Can you work these out from the model? Positions are in its coordinate system, mm. Face numbers are marked on the shaded views. A direction names the side the tool comes from. Give positions to 0.01 mm unless a question says otherwise; leave off trailing zeros. Loops run counter-clockwise (first coordinate to the right, second up) from the corner with the lowest first, then second, coordinate; pieces in that order, holes last. Notation, with made-up numbers: (-39.5, 1) -> (-1.5, 1) arc R26 ccw to (-1.5, 39) -> close; hole circle Ø2 at (36.5, 17.25). An arc over 180 degrees is marked (long way). Return JSON: item names as keys, results as strings. Group by question number.
Q1. Suppose I cut it at B-B, the plane z = -5. Please give me the cut outline in (x, y).
Q2. Suppose I cut it at D-D, the plane x = -13.5. Please give me the cut outline in (y, z).
Q3. I need wall thicknesses on line 1 along Y through (x, z) = (-4, -3); line 2 along X through (y, z) = (-8.45, -5); line 3 along Z through (x, y) = (27.5, -3). Which ranges of each line are inside material? Lowest first, please. Write a range as [from, to].
Q4. Suppose I cut it at C-C, the plane y = -4.5. Please give me the cut outline in (x, z).
Q5. Which directions (+Z, -Z, +X, -X, +Y, -Y) give clear straight access to the entire face, cutting with the end or side of a thin tool? Please do the marked faces 1 and 2.
Q6. Suppose I cut it at A-A, the plane x = -50. Please give me the cut outline in (y, z).
Q7. Will these pins go through, and if not, where does the flat tip stop? pin 1 (1 mm diameter, centred on x = 32.5, z = -0.5, fed in from +Y); pin 2 (0.6 mm diameter, centred on x = 60, y = -0.5, fed in from +Z); pin 3 (2.5 mm diameter, centred on x = 0, z = -5, fed in from -Y); pin 4 (5 mm diameter, centred on y = -6, z = -2.5, fed in from +X).
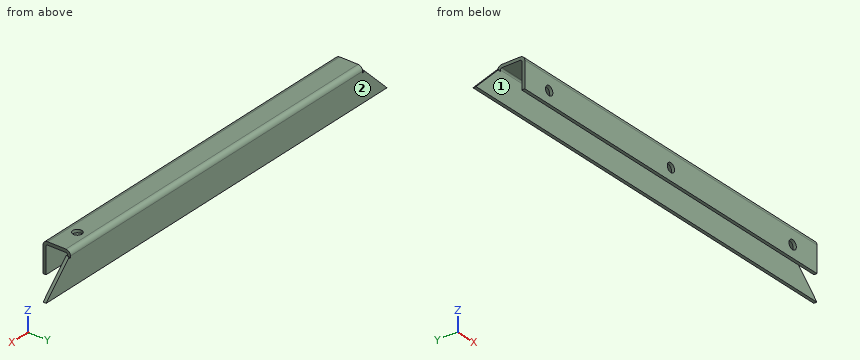
```python
from build123d import *

# Parameters (mm, degrees)
BASE_FLANGE1_DEPTH            = 1
EDGE_FLANGE1_STRIP_W          = 5
EDGE_FLANGE1_STRIP_H          = 1
EDGE_FLANGE1_STRIP_CUT_DEPTH  = 120
EDGE_FLANGE1_RELIEF_W         = 5.5
EDGE_FLANGE1_RELIEF_H         = 0.5
EDGE_FLANGE1_RELIEF_CUT_DEPTH = 1
EDGE_FLANGE1_DEPTH            = 120
EDGE_FLANGE2_STRIP_W          = 5
EDGE_FLANGE2_STRIP_H          = 1
EDGE_FLANGE2_STRIP_CUT_DEPTH  = 120
EDGE_FLANGE2_DEPTH            = 120
SKETCH12_R                    = 1.5
CUT_EXTRUDE1_DEPTH            = 3
SKETCH13_R                    = 1.5
CUT_EXTRUDE2_DEPTH            = 3


# Sheet-metal steps are written as plain solids
with BuildPart() as part:
    # Sketch1 → Base-Flange1 (new body)
    with BuildSketch(Plane(origin=(0, 0, 0), x_dir=(1, 0, 0), z_dir=(0, 1, 0))):
        Polygon((-60, 0), (60, 0), (70, 10), (-70, 10), align=None)
    extrude(amount=-BASE_FLANGE1_DEPTH)

    # Edge-Flange1 strip (across the edge) → Edge-Flange1 strip cut (cut)
    with BuildSketch(Plane(origin=(60, -1, 0), x_dir=(0, 0, -1), z_dir=(-1, 0, 0))):
        with Locations((-2, -0.5)):
            Rectangle(EDGE_FLANGE1_STRIP_W, EDGE_FLANGE1_STRIP_H)
    extrude(amount=EDGE_FLANGE1_STRIP_CUT_DEPTH, mode=Mode.SUBTRACT)

    # Edge-Flange1 relief (on the sheet) → Edge-Flange1 relief cut (cut)
    with BuildSketch(Plane(origin=(60, -1, -0.5), x_dir=(0, 0, -1), z_dir=(0, -1, 0))):
        with Locations((-2.25, 0.25)):
            Rectangle(EDGE_FLANGE1_RELIEF_W, EDGE_FLANGE1_RELIEF_H)
        with Locations((-2.25, -120.25)):
            Rectangle(EDGE_FLANGE1_RELIEF_W, EDGE_FLANGE1_RELIEF_H)
    extrude(amount=-EDGE_FLANGE1_RELIEF_CUT_DEPTH, mode=Mode.SUBTRACT)

    # Edge-Flange1 section (across the edge) → Edge-Flange1 (add)
    with BuildSketch(Plane(origin=(60, -1, 0), x_dir=(0, 0, -1), z_dir=(-1, 0, 0))):
        with BuildLine():
            Line((-1, 0.5), (-1, 7))
            Line((-1, 7), (0, 7))
            Line((0, 7), (0, 0.5))
            ThreePointArc((0, 0.5), (0.146446609, 0.146446609), (0.5, 0))
            Line((0.5, 0), (0.5, -1))
            ThreePointArc((0.5, -1), (-0.560660172, -0.560660172), (-1, 0.5))
        make_face()
    extrude(amount=EDGE_FLANGE1_DEPTH)

    # Edge-Flange2 strip (across the edge) → Edge-Flange2 strip cut (cut)
    with BuildSketch(Plane(origin=(60, -8, 0), x_dir=(0, 1, 0), z_dir=(-1, 0, 0))):
        with Locations((-2, -0.5)):
            Rectangle(EDGE_FLANGE2_STRIP_W, EDGE_FLANGE2_STRIP_H)
    extrude(amount=EDGE_FLANGE2_STRIP_CUT_DEPTH, mode=Mode.SUBTRACT)

    # Edge-Flange2 section (across the edge) → Edge-Flange2 (add)
    with BuildSketch(Plane(origin=(60, -8, 0), x_dir=(0, 1, 0), z_dir=(-1, 0, 0))):
        with BuildLine():
            Line((-1, 0.5), (-1, 9))
            Line((-1, 9), (0, 9))
            Line((0, 9), (0, 0.5))
            ThreePointArc((0, 0.5), (0.146446609, 0.146446609), (0.5, 0))
            Line((0.5, 0), (0.5, -1))
            ThreePointArc((0.5, -1), (-0.560660172, -0.560660172), (-1, 0.5))
        make_face()
    extrude(amount=EDGE_FLANGE2_DEPTH)

    # Sketch12 → Cut-Extrude1 (cut)
    with BuildSketch(Plane.XZ.offset(9)):
        with Locations(Location((-50, -5, 0), (0, 0, 270))):
            Circle(SKETCH12_R)
        with Locations(Location((0, -5, 0), (0, 0, 270))):
            Circle(SKETCH12_R)
        with Locations(Location((50, -5, 0), (0, 0, 270))):
            Circle(SKETCH12_R)
    extrude(amount=-CUT_EXTRUDE1_DEPTH, mode=Mode.SUBTRACT)

    # Sketch13 → Cut-Extrude2 (cut)
    with BuildSketch(Plane(origin=(0, 0, 0), x_dir=(-1, 0, 0), z_dir=(0, 0, -1))):
        with Locations(Location((-51.5, -4.5, 0), (0, 0, 90))):
            Circle(SKETCH13_R)
    extrude(amount=-CUT_EXTRUDE2_DEPTH, mode=Mode.SUBTRACT)


solid = part.part
```
Ans:
{
 "1": {"outline": "(-65, -1) -> (65, -1) -> (65, 0) -> (-65, 0) -> close; (-60, -9) -> (-51.5, -9) -> (-51.5, -8) -> (-60, -8) -> close; (-48.5, -9) -> (-1.5, -9) -> (-1.5, -8) -> (-48.5, -8) -> close; (1.5, -9) -> (48.5, -9) -> (48.5, -8) -> (1.5, -8) -> close; (51.5, -9) -> (60, -9) -> (60, -8) -> (51.5, -8) -> close"},
 "2": {"outline": "(-9, -9) -> (-8, -9) -> (-8, -0.5) arc R0.5 cw to (-7.5, 0) -> (-1.5, 0) arc R0.5 cw to (-1, -0.5) -> (-1, -10) -> (0, -10) -> (0, -0.5) arc R1.5 ccw to (-1.5, 1) -> (-7.5, 1) arc R1.5 ccw to (-9, -0.5) -> close"},
 "3": {"line 1": "y = [-9, -8], [-1, 0]", "line 2": "x = [-60, -51.5], [-48.5, -1.5], [1.5, 48.5], [51.5, 60]", "line 3": "z = [0, 1]"},
 "4": {"outline": "(-60, 0) -> (50, 0) -> (50, 1) -> (-60, 1) -> close; (53, 0) -> (60, 0) -> (60, 1) -> (53, 1) -> close"},
 "5": {"face 1": "-Z, +X, -X", "face 2": "+Z, -Z, +X, -X, +Y"},
 "6": {"outline": "(-9, -9) -> (-8, -9) -> (-8, -6.5) -> (-9, -6.5) -> close; (-9, -3.5) -> (-8, -3.5) -> (-8, -0.5) arc R0.5 cw to (-7.5, 0) -> (-1.5, 0) arc R0.5 cw to (-1, -0.5) -> (-1, -10) -> (0, -10) -> (0, -0.5) arc R1.5 ccw to (-1.5, 1) -> (-7.5, 1) arc R1.5 ccw to (-9, -0.5) -> close"},
 "7": {"pin 1": "stops at y = 0", "pin 2": "stops at z = 0.83", "pin 3": "stops at y = -1", "pin 4": "stops at x = 60"}
}
